Could you check a few things on this model? Use its own coordinates, in mm. A direction names the side the tool comes from. Round coordinates to 2 decimals unless told otherwise and drop trailing zeros. Loops run counter-clockwise (first coordinate to the right, second up) from the corner with the lowest first, then second, coordinate; pieces in that order, holes last. Notation, with made-up numbers: (61, 14.5) -> (73, 14.5) arc R4 cw to (73, 18.5) -> close; hole circle Ø10 at (61.25, -15.75). An arc over 180 degrees is marked (long way). Write each question's results on one line, items separated by ' | '. Start each with the question number.
1) Imagine slicing it at B-B, the plane y = 7. List the corners of the cut face in (x, z) for me.
2) Which directions (+Z, -Z, +X, -X, +Y, -Y) give clear straight access to the entire face, cutting with the end or side of a thin tool? Please do faces 4 (the flat face through (16, 17, 84.5)), 5 (the flat face through (80, 24, 15)), 6 (the flat face through (32, 0, 48)).
3) If I drill on probe 1 along X at (y, z) = (1, 80); probe 2 along X at (y, z) = (1.5, 10.8); probe 3 along X at (y, z) = (1.15, 5.4), over which ranges is the centre line in solid material (lowest first)?
4) We'd pull the mould along X, two halves only. Please class faces 1 (the flat face through (15, 42, 21)), 2 (the flat face through (95, 24, 53)), 3 (the cylindrical face through (4.13, 21.72, 26.65)): pulls with the +X half, pulls with the -X half, needs draft (parallel to the pull), parting line crosses it, or undercut.
5) Imagine slicing it at C-C, the plane x = 15. List the corners of the cut face in (y, z) for me, plus the area to 3 significant figures.
6) Imagine slicing it at D-D, the plane z = 80. List the corners of the cut face in (x, y) for me, plus the area to 3 significant figures.
7) For P1, Ø1.6, axis at x = 46, y = 1.5, coming from the +Z side; P2, Ø12, axis at x = 9.5, y = 5, coming from the +Z side; P3, Ø0.6, axis at y = 0.5, z = 94.5, coming from the +X side; P4, Ø19.5, axis at x = 31.5, z = 26, coming from the -Y side, each with a flat end and sliding along its axis, tell me the tip position at first contact or that it passes through.
8) Imagine slicing it at A-A, the plane z = 5.4. List the corners of the cut face in (x, y) for me, plus the area to 3 significant figures.
from build123d import *

# Parameters (mm, degrees)
SKETCH1_W           = 65
SKETCH1_H           = 98
SKETCH1_R           = 1.75
SKETCH1_W_2         = 5.703642488
SKETCH1_H_2         = 7.830424434
SKETCH1_H_3         = 8.120440153
BOSS_EXTRUDE1_DEPTH = 2
SKETCH2_W           = 15
SKETCH2_H           = 6
BOSS_EXTRUDE2_DEPTH = 10
SKETCH3_R           = 12.25
BOSS_EXTRUDE3_DEPTH = 40
SKETCH4_W           = 30
SKETCH4_H           = 13
BOSS_EXTRUDE4_DEPTH = 30
SKETCH5_W           = 30
SKETCH5_H           = 11
BOSS_EXTRUDE5_DEPTH = 10
SKETCH6_W           = 30
SKETCH6_H           = 78
BOSS_EXTRUDE6_DEPTH = 45.5
SKETCH7_W           = 30
SKETCH7_H           = 78
BOSS_EXTRUDE7_DEPTH = 2.1


with BuildPart() as part:
    # Sketch1 → Boss-Extrude1 (new body)
    with BuildSketch(Plane(origin=(0, 0, 0), x_dir=(1, 0, 0), z_dir=(0, 1, 0))):
        with Locations((32.5, -49)):
            Rectangle(SKETCH1_W, SKETCH1_H)
        with Locations(Location((4.8, -5.4, 0), (0, 0, 270))):
            Circle(SKETCH1_R, mode=Mode.SUBTRACT)
        with Locations(Location((59.2, -10.8, 0), (0, 0, 270))):
            Circle(SKETCH1_R, mode=Mode.SUBTRACT)
        with Locations(Location((19.5, -80, 0), (0, 0, 270))):
            Circle(SKETCH1_R, mode=Mode.SUBTRACT)
        with Locations(Location((47.5, -80.1, 0), (0, 0, 270))):
            Circle(SKETCH1_R, mode=Mode.SUBTRACT)
        with Locations((57.239046226, -41.024145722)):
            Rectangle(SKETCH1_W_2, SKETCH1_H_2, mode=Mode.SUBTRACT)
        with Locations((57.239046226, -70.750756999)):
            Rectangle(SKETCH1_W_2, SKETCH1_H_3, mode=Mode.SUBTRACT)
    extrude(amount=BOSS_EXTRUDE1_DEPTH)

    # Sketch2 → Boss-Extrude2 (add)
    with BuildSketch(Plane(origin=(0, 2, 0), x_dir=(1, 0, 0), z_dir=(0, 1, 0))):
        with Locations((21, -1)):
            Rectangle(SKETCH2_W, SKETCH2_H)
    extrude(amount=BOSS_EXTRUDE2_DEPTH)

    # Sketch3 → Boss-Extrude3 (add)
    with BuildSketch(Plane(origin=(0, 2, 0), x_dir=(1, 0, 0), z_dir=(0, 1, 0))):
        with Locations(Location((15, -21, 0), (0, 0, 270))):
            Circle(SKETCH3_R)
        with Locations(Location((40, -21, 0), (0, 0, 270))):
            Circle(SKETCH3_R)
    extrude(amount=BOSS_EXTRUDE3_DEPTH)

    # Sketch4 → Boss-Extrude4 (add)
    with BuildSketch(Plane(origin=(0, 2, 0), x_dir=(1, 0, 0), z_dir=(0, 1, 0))):
        with Locations((16, -91)):
            Rectangle(SKETCH4_W, SKETCH4_H)
    extrude(amount=BOSS_EXTRUDE4_DEPTH)

    # Sketch5 → Boss-Extrude5 (add)
    with BuildSketch(Plane(origin=(0, 2, 0), x_dir=(1, 0, 0), z_dir=(0, 1, 0))):
        with Locations((47.2, -93)):
            Rectangle(SKETCH5_W, SKETCH5_H)
    extrude(amount=BOSS_EXTRUDE5_DEPTH)



with BuildPart() as body_2:
    # Sketch6 → Boss-Extrude6 (new body)
    with BuildSketch(Plane(origin=(0, 2, 0), x_dir=(1, 0, 0), z_dir=(0, 1, 0))):
        with Locations((80, -54)):
            Rectangle(SKETCH6_W, SKETCH6_H)
    extrude(amount=BOSS_EXTRUDE6_DEPTH)


with BuildPart() as part_1:
    add(part.part)

    add(body_2.part)  # Boss-Extrude7 merges body 2
    # Sketch7 → Boss-Extrude7 (add)
    with BuildSketch(Plane.XZ.offset(-2)):
        with Locations((80, 54)):
            Rectangle(SKETCH7_W, SKETCH7_H)
    extrude(amount=BOSS_EXTRUDE7_DEPTH)


solid = part_1.part
Checked values:
1) outline: (1, 84.5) -> (31, 84.5) -> (31, 97.5) -> (1, 97.5) -> close; circle Ø24.5 at (15, 21); (13.5, -2) -> (28.5, -2) -> (28.5, 4) -> (13.5, 4) -> close; circle Ø24.5 at (40, 21); (32.2, 87.5) -> (62.2, 87.5) -> (62.2, 98.5) -> (32.2, 98.5) -> close; (65, 15) -> (95, 15) -> (95, 93) -> (65, 93) -> close
2) face 4: -X, +Y | face 5: -Z, +X, +Y, -Y | face 6: +Z, -Z, -X, -Y
3) probe 1: 0 to 17.75, 21.25 to 45.75, 49.25 to 95 | probe 2: 0 to 57.45, 60.95 to 65 | probe 3: 0 to 3.05, 6.55 to 65
4) face 1: needs draft | face 2: pulls with the +X half | face 3: undercut
5) outline: (0, 0) -> (2, 0) -> (2, -2) -> (12, -2) -> (12, 4) -> (2, 4) -> (2, 8.75) -> (42, 8.75) -> (42, 33.25) -> (2, 33.25) -> (2, 84.5) -> (32, 84.5) -> (32, 97.5) -> (2, 97.5) -> (2, 98) -> (0, 98) -> close | area: 1,630 mm^2
6) outline: (0, 0) -> (17.75, 0) -> (17.75, 2) -> (0, 2) -> close; (21.25, 0) -> (45.75, 0) -> (45.75, 2) -> (21.25, 2) -> close; (49.25, 0) -> (65, 0) -> (65, -0.1) -> (95, -0.1) -> (95, 47.5) -> (65, 47.5) -> (65, 2) -> (49.25, 2) -> close | area: 1,540 mm^2
7) P1: z = 98.5 | P2: z = 98 | P3: x = 65 | P4: y = 0
8) outline: (0, 0) -> (3.05, 0) -> (3.05, 2) -> (0, 2) -> close; (6.55, 0) -> (65, 0) -> (65, 2) -> (6.55, 2) -> close | area: 123 mm^2
